Check sheet for the modelled part. Datum: model origin and axes. Units: mm. A direction names the side the tool comes from. Round coordinates to 2 decimals unless told otherwise and drop trailing zeros. Order: outer loops, then holes, each group sorted by start corner. A loop starts at its lowest first (then second) coordinate and runs counter-clockwise, first axis right, second up. Notation, with made-up numbers: (-35.75, 46.25) -> (8.25, 46.25) arc R17 cw to (8.25, 65.25) -> close; hole circle Ø9 at (60, 36). An arc over 180 degrees is marked (long way). Answer in a Markdown table with one row per item.
```python
from build123d import *

# Parameters (mm, degrees)
SKETCH1_R              = 64
SKETCH1_R_2            = 60
RIM_DEPTH              = 28
SKETCH2_R              = 65.5
SKETCH2_R_2            = 63
INNER_BEAD_LIP_DEPTH   = 1.5
SKETCH3_R              = 65.5
SKETCH3_R_2            = 63
OUTER_BEAD_LIP_DEPTH   = 1.5
SKETCH4_R              = 61
WEB_DEPTH              = 7
SKETCH5_R              = 8
HUB_BOSS_DEPTH         = 24
SKETCH6_R              = 13
LIGHTENING_HOLES_DEPTH = 9
D_BORE_4MM_DEPTH       = 30
SKETCH9_R              = 69
SKETCH9_R_2            = 64
BED_RING_DEPTH         = 1.5
SKETCH10_R             = 1.3
GRUB_SCREW_M3_DEPTH    = 9
SKETCH11_R             = 1.9
GRUB_KEY_ACCESS_DEPTH  = 62.5


with BuildPart() as part:
    # Sketch1 → Rim (new body)
    with BuildSketch(Plane.XY):
        Circle(SKETCH1_R)
        Circle(SKETCH1_R_2, mode=Mode.SUBTRACT)
    extrude(amount=RIM_DEPTH)

    # Sketch2 → Inner_bead_lip (add)
    with BuildSketch(Plane.XY):
        Circle(SKETCH2_R)
        Circle(SKETCH2_R_2, mode=Mode.SUBTRACT)
    extrude(amount=INNER_BEAD_LIP_DEPTH)

    # Sketch3 → Outer_bead_lip (add)
    with BuildSketch(Plane.XY.offset(26.5)):
        Circle(SKETCH3_R)
        Circle(SKETCH3_R_2, mode=Mode.SUBTRACT)
    extrude(amount=OUTER_BEAD_LIP_DEPTH)

    # Sketch4 → Web (add)
    with BuildSketch(Plane.XY):
        Circle(SKETCH4_R)
    extrude(amount=WEB_DEPTH)

    # Sketch5 → Hub_boss (add)
    with BuildSketch(Plane.XY):
        Circle(SKETCH5_R)
    extrude(amount=HUB_BOSS_DEPTH)

    # Sketch6 → Lightening_holes (cut)
    with BuildSketch(Plane.XY.offset(-1)):
        with Locations((32.04293994, 18.5)):
            Circle(SKETCH6_R)
        with Locations((0, 37)):
            Circle(SKETCH6_R)
        with Locations((-32.04293994, 18.5)):
            Circle(SKETCH6_R)
        with Locations((-32.04293994, -18.5)):
            Circle(SKETCH6_R)
        with Locations((0, -37)):
            Circle(SKETCH6_R)
        with Locations((32.04293994, -18.5)):
            Circle(SKETCH6_R)
    extrude(amount=LIGHTENING_HOLES_DEPTH, mode=Mode.SUBTRACT)

    # Sketch7 → D_bore_4mm (cut)
    with BuildSketch(Plane.XY.offset(-1)):
        with BuildLine():
            Line((1.5, -1.397318861), (1.5, 1.397318861))
            ThreePointArc((1.5, 1.397318861), (-2.05, 0), (1.5, -1.397318861))
        make_face()
    extrude(amount=D_BORE_4MM_DEPTH, mode=Mode.SUBTRACT)

    # Sketch8 → Tyre (revolve)
    with BuildSketch(Plane(origin=(0, 0, 0), x_dir=(0, 0, -1), z_dir=(1, 0, 0)), mode=Mode.PRIVATE) as tyre_sk:
        Polygon((-1.5, 64), (-26.5, 64), (-26.5, 69), (-25.5, 70), (-19, 70), (-19, 68.8), (-17, 68.8), (-17, 70), (-11, 70), (-11, 68.8), (-9, 68.8), (-9, 70), (-2.5, 70), (-1.5, 69), align=None)
    revolve(tyre_sk.sketch.rotate(Axis((0, 0, 0), (0, 0, 1)), 90), axis=Axis((0, 0, 0), (0, 0, 1)))

    # Sketch9 → Bed_ring (add)
    with BuildSketch(Plane.XY):
        with Locations(Location((0, 0, 0), (0, 0, 180))):
            Circle(SKETCH9_R)
        Circle(SKETCH9_R_2, mode=Mode.SUBTRACT)
    extrude(amount=BED_RING_DEPTH)

    # Sketch10 → Grub_screw_M3 (cut)
    with BuildSketch(Plane(origin=(0, 0, 0), x_dir=(0, 0, -1), z_dir=(1, 0, 0))):
        with Locations(Location((-3.6, 0, 0), (0, 0, 270))):
            Circle(SKETCH10_R)
    extrude(amount=GRUB_SCREW_M3_DEPTH, mode=Mode.SUBTRACT)

    # Sketch11 → Grub_key_access (cut)
    with BuildSketch(Plane(origin=(8.5, 0, 0), x_dir=(0, 0, -1), z_dir=(1, 0, 0))):
        with Locations(Location((-3.6, 0, 0), (0, 0, 54.623459848))):
            Circle(SKETCH11_R)
    extrude(amount=GRUB_KEY_ACCESS_DEPTH, mode=Mode.SUBTRACT)


solid = part.part
```
(1) Tool access check on faces 1 (the cylindrical face through (38.82, -0.261, 1.718)), 2 (the flat face through (52, 46, 9)), 3 (the cylindrical face through (-1.73, -7.81, 15.38)). Record the directions out of +Z, -Z, +X, -X, +Y, -Y that give a thin tool (end or side, any length) a straight path to the whole face; none if there is none.
Solutions:
| item | result |
|---|---|
| face 1 | +X |
| face 2 | none |
| face 3 | +Z |
(2) Section check A-A on z = 13.5. Record the boundary of the cut face in (x, y), plus the area to 3 significant figures.
Solutions:
| item | result |
|---|---|
| outline | circle Ø140 at (0, 0); circle Ø16 at (0, 0); hole circle Ø120 at (0, 0); hole (1.5, -1.4) -> (1.5, 1.4) arc R2.05 ccw (long way) to start |
| area | 4,270 mm^2 |
(3) Draft check along Z on faces 4 (the flat face through (-52, 46, 19)), 5 (the cylindrical face through (68.933, -3.034, 0.74)), 6 (the flat face through (61, 25, 26.5)). Enter one of: pulls with the +Z half, pulls with the -Z half, needs draft (parallel to the pull), parting line crosses it, or undercut.
Solutions:
| item | result |
|---|---|
| face 4 | undercut |
| face 5 | needs draft |
| face 6 | pulls with the +Z half |
(4) Scan lines: probe 1 along Y at (x, z) = (0, 1.5); probe 2 along X at (y, z) = (-36, 5.75); probe 3 along X at (y, z) = (-18.5, 2). Record each from-to range of solid material in increasing order. Write a range as from..to.
Solutions:
| item | result |
|---|---|
| probe 1 | -69..-50, -24..-2.05, 2.05..24, 50..69 |
| probe 2 | -60.03..-12.96, 12.96..60.03 |
| probe 3 | -66.99..-45.04, -19.04..19.04, 45.04..66.99 |
(5) Section check B-B on x = 26. Give the number of separate pieces and of enclosed holes in the cut face, plus the area to 3 significant figures.
Solutions:
| item | result |
|---|---|
| separate pieces | 3 |
| enclosed holes | 1 |
| area | 1,000 mm^2 |
(6) Depth check by flat-ended pin: pin 1 Ø1 at (x, z) = (-1.5, 23.5) entering from -Y; pin 2 Ø13 at (x, y) = (-2.5, -1.5) entering from +Z; pin 3 Ø5 at (y, z) = (34.5, 14) entering from -X; pin 4 Ø6 at (x, y) = (-35, 11.5) entering from -Z. Enter the tip coordinate at first touch or a pass-through.
Solutions:
| item | result |
|---|---|
| pin 1 | y = -69.99 |
| pin 2 | z = 24 |
| pin 3 | x = -62.26 |
| pin 4 | through |
